Autodesk Inventor part; units mm, degrees
ref_plane "YZ Plane" through (0, 0, 0) normal (1, 0, 0) x (0, 1, 0)
ref_plane "XZ Plane" through (0, 0, 0) normal (0, 1, 0) x (-1, 0, 0)
ref_plane "XY Plane" through (0, 0, 0) normal (0, 0, 1) x (1, 0, 0)
sketch "Szkic2" plane through (0, 0, 0) normal (0, 1, 0) x (-1, 0, 0)
  line L0 (0, 0) -> (-190, 0)
  line L1 (-190, 0) -> (-190, 270)
  line L2 (-190, 270) -> (0, 270)
  line L3 (0, 270) -> (0, 0)
  dimension "d0" = 190
  dimension "d1" = 270
extrude "Wyciągnięcie proste1" add sketch "Szkic2" along normal mid plane 10
fillet "Zaokrąglenie1" radius 4 4 edges at (190, 0, 0) (0, 0, 0) (0, 0, 270) (190, 0, 270)
sketch "Szkic4" plane through (0, 0, 0) normal (0, 1, 0) x (-1, 0, 0)
  line L0 (-4, 4) -> (-186, 4)
  line L1 (-186, 4) -> (-186, 266)
  line L2 (-186, 266) -> (-4, 266)
  line L3 (-4, 266) -> (-4, 4)
  line L4 (-186, 0) -> (-4, 0)
  line L5 (0, 4) -> (0, 266)
  line L6 (-190, 266) -> (-190, 4)
  line L7 (-4, 270) -> (-186, 270)
  point P0 (0, 0)
  dimension "d13" = 4
  dimension "d14" = 4
  dimension "d16" = 4
  dimension "d17" = 4
extrude "Wyciągnięcie proste3" cut sketch "Szkic4" against normal blind 5
properties part number "klapka1"
Input: part model. Units: mm. Frame: model coordinates. A direction names the side the tool comes from. Coordinates: 2 decimals unless noted, no trailing zeros. Loops run counter-clockwise (first coordinate to the right, second up) from the corner with the lowest first, then second, coordinate; pieces in that order, holes last.
(1) First-contact query: pin 1 Ø5 at (y, z) = (-2.5, 123.5) entering from -X. Flat tip, straight axial feed; report the tip coordinate or a pass-through.
(2) Set-up query: faces 4 (the face through (186, -2, 133)), 5 (the face through (96, 5, 137)). Return all of +Z, -Z, +X, -X, +Y, -Y with unobstructed straight access to the full face (end or side cutting, diameter ignored); none if empty.
(3) Pull-direction query (X, two-part tool) for faces 1 (the face through (190, 0, 133)), 2 (the face through (96, -2, 266)), 3 (the face through (96, 0, 270)); classes: released by +X, released by -X, zero draft, split by the parting line, or undercut.
(4) Section A-A on y = -2.25. Return the cut outline in (x, z).
(5) Material intervals for probe 1 along X at (y, z) = (-1.25, 217); probe 2 along Z at (x, y) = (118.5, -3.25); probe 3 along Y at (x, z) = (24, 175), sorted ascending.
(6) Section B-B on z = 231.5. Return the cut outline in (x, y), then the cut area to 3 significant figures.
(7) Section C-C on x = 105. Return the cut outline in (y, z).
Data:
1. pin 1: stops at x = 0
2. face 4: -Y
2. face 5: +Z, -Z, +X, -X, +Y
3. face 1: released by +X
3. face 2: undercut
3. face 3: zero draft
4. outline: (0, 4) arc R4 ccw to (4, 0) - (186, 0) arc R4 ccw to (190, 4) - (190, 266) arc R4 ccw to (186, 270) - (4, 270) arc R4 ccw to (0, 266) - close; hole (4, 4) - (186, 4) - (186, 266) - (4, 266) - close
5. probe 1: x = 0 to 4, 186 to 190
5. probe 2: z = 0 to 4, 266 to 270
5. probe 3: y = 0 to 5
6. outline: (0, -5) - (4, -5) - (4, 0) - (186, 0) - (186, -5) - (190, -5) - (190, 5) - (0, 5) - close
6. area: 990 mm2
7. outline: (-5, 0) - (5, 0) - (5, 270) - (-5, 270) - (-5, 266) - (0, 266) - (0, 4) - (-5, 4) - close
